Check sheet for the modelled part. Datum: model origin and axes. Units: mm. A direction names the side the tool comes from. Give positions to 0.01 mm unless a question says otherwise; leave off trailing zeros. Order: outer loops, then holes, each group sorted by start corner. A loop starts at its lowest first (then second) coordinate and runs counter-clockwise, first axis right, second up.
```python
from build123d import *

# Parameters (mm, degrees)
F3_D     = 1.95
F3_DEPTH = 8.75
F3_TIP   = 0.5858391036


with BuildPart() as f1:
    # F0 (on Front) → F1 (revolve)
    with BuildSketch(Plane.XZ):
        with BuildLine():
            Line((0, -18.5), (0, 0))
            Line((0, 0), (0, 58))
            Line((0, 58), (-5.5, 58))
            Line((-5.5, 58), (-5.5, 56.75))
            Line((-5.5, 56.75), (-6.5, 56.75))
            Line((-6.5, 56.75), (-6.5, 41.6852130745))
            Line((-6.5, 41.6852130745), (-5.5, 41.6852130745))
            Line((-5.5, 41.6852130745), (-4.25, 33.6852130745))
            Line((-4.25, 33.6852130745), (-3, 33.6852130745))
            Line((-3, 33.6852130745), (-3, 7.6852130745))
            ThreePointArc((-3, 7.6852130745), (-8.245736984, -0.2651821852), (-2.5, -7.8620925968))
            Line((-2.5, -7.8620925968), (-2.5, -18.5))
            Line((-2.5, -18.5), (0, -18.5))
        make_face()
    revolve(axis=Axis((0, 0, 29), (0, 0, 1)))

    # F3 (one way)
    with BuildSketch(Plane(origin=(0, 0, 0), x_dir=(0, 1, 0), z_dir=(-1, 0, 0))):
        with Locations((0, 0)):
            Circle(F3_D / 2)
    extrude(amount=-F3_DEPTH, mode=Mode.SUBTRACT)
    with Locations(Plane(origin=(0, 0, 0), x_dir=(0, 1, 0), z_dir=(-1, 0, 0))):
        with Locations((0, 0)):
            with Locations((0, 0, -(F3_DEPTH + F3_TIP / 2))):  # 118° drill point
                Cone(0, F3_D / 2, F3_TIP, mode=Mode.SUBTRACT)


solid = f1.part
```
(1) Cross-section at B-B on z = 33. Enter the section's corners in (x, y), then the cut area to 3 significant figures.
Response values:
outline: circle Ø6 at (0, 0)
area: 28.3 mm2
(2) Cross-section at D-D on z = 42.5. Enter the section's corners in (x, y).
Response values:
outline: circle Ø13 at (0, 0)
(3) Cross-section at A-A on y = 0. Enter the section's corners in (x, z) (3 decimals), then the cut area to 3 significant figures.
Response values:
outline: (-6.5, 41.685) - (-5.5, 41.685) - (-4.25, 33.685) - (-3, 33.685) - (-3, 7.685) arc R8.25 ccw to (-2.5, -7.862) - (-2.5, -18.5) - (2.5, -18.5) - (2.5, -7.862) arc R8.25 ccw to (8.192, -0.975) - (0, -0.975) - (0, 0.975) - (8.192, 0.975) arc R8.25 ccw to (3, 7.685) - (3, 33.685) - (4.25, 33.685) - (5.5, 41.685) - (6.5, 41.685) - (6.5, 56.75) - (5.5, 56.75) - (5.5, 58) - (-5.5, 58) - (-5.5, 56.75) - (-6.5, 56.75) - close
area: 691 mm2
(4) Material ranges on L1, parallel to Z at x = 1.75, y = 0 (3 decimals); L2, parallel to Z at x = 6.25, y = 0 (3 decimals); L3, parallel to Z at x = 6, y = 0 (3 decimals), recorded low to high.
Response values:
L1: z = -18.5 to -0.975, 0.975 to 58
L2: z = -5.385 to -0.975, 0.975 to 5.385, 41.685 to 56.75
L3: z = -5.662 to -0.975, 0.975 to 5.662, 41.685 to 56.75
(5) Gauge pin test, flat ends, axial feed: pin 1 Ø1.6 at (y, z) = (-0.5, 0.5) entering from +X; pin 2 Ø2 at (y, z) = (2.5, 17) entering from +X; pin 3 Ø5 at (y, z) = (4.5, -3) entering from -X; pin 4 Ø5 at (x, z) = (-4, 2.5) entering from -Y. Record the tip position at first contact, or that the pin passes through.
Response values:
pin 1: stops at x = 8.19
pin 2: stops at x = 2.6
pin 3: stops at x = -7.72
pin 4: stops at y = -7.95
(6) Cross-section at C-C on z = 0. Enter the section's corners in (x, y) (3 decimals).
Response values:
outline: (0, -0.975) - (0, 0.975) - (8.192, 0.975) arc R8.25 ccw (long way) to (8.192, -0.975) - close
(7) Release check for a two-part mould opening along Z. For faces 5 (the face through (0, 0, 0)), 6 (the face through (-5, -3, 56.75)), 7 (the face through (5.158, 3.955, 49.112)) record: released by +Z, released by -Z, zero draft, split by the parting line, or undercut.
Response values:
face 5: undercut
face 6: released by +Z
face 7: zero draft
(8) Set-up check for faces 1 (the face through (1.19, 5.37, 57.37)), 2 (the face through (4.04, -0.72, -0.66)), 3 (the face through (0.54, 2.44, -13.26)), 4 (the face through (3, 0, 21)): record each of +Z, -Z, +X, -X, +Y, -Y from which the full face is reachable in a straight line by a thin tool's end or side.
Response values:
face 1: +Z
face 2: +X
face 3: -Z
face 4: none
